Read the model definition and answer for the solid it produces. Units are mm, in the model's axes. Face numbers are marked on the shaded views. Coordinates: 2 decimals unless noted, no trailing zeros. Write each loop counter-clockwise with the first axis right and the second up, starting at its lowest first coordinate (ties: lowest second). Pieces come first, ordered by that corner, then holes. Notation, with made-up numbers: (33.25, 28) -> (54.25, 28) arc R21 ccw to (54.25, 66) -> close; hole circle Ø7 at (75.25, -40). An arc over 180 degrees is marked (long way). Answer in a Markdown table with one row per item. Add a question column.
Item 1: Section A-A on x = 0 is taken. Write down the section's boundary in (y, z).
Item 2: Given pin 1 Ø1 at (x, z) = (-9.5, 11) entering from +Y; pin 2 Ø3.5 at (x, y) = (0, -8) entering from +Z; pin 3 Ø5 at (x, z) = (-3, 8) entering from -Y, each flat-ended and moving along its own axis, determine where each tip first touches the part or whether it passes through.
Item 3: Straight lines are drawn through the part: line 1 (Y direction, x = 0, z = 11); line 2 (X direction, y = -9, z = 13); line 3 (Y direction, x = -13, z = 11). For each, find the intervals that lie inside material, in ascending order. Write a range as from..to.
Item 4: For a pull along X with two mould halves and no side action, classify the marked faces 1, 2 and 3 as +X half, -X half, draft (parallel to the pull), parting line (faces both ways), or undercut.
Item 5: Section B-B on z = 8.5 is taken. Write down the section's boundary in (x, y), then the cut area to 3 significant figures.
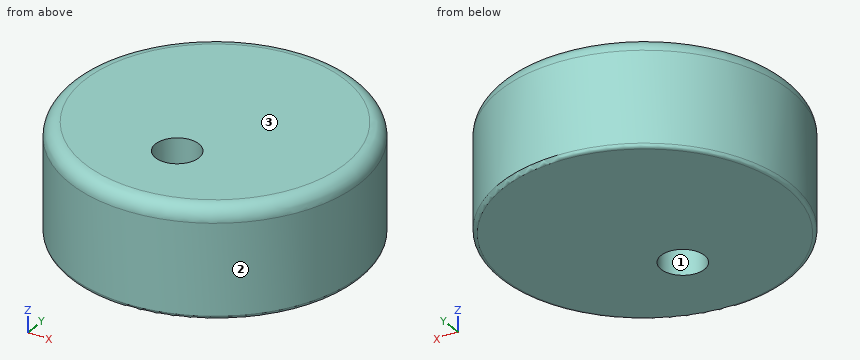
```python
from build123d import *

# Parameters (mm, degrees)
SKETCH1_R           = 20
BOSS_EXTRUDE1_DEPTH = 15
SKETCH2_R           = 3
CUT_EXTRUDE1_DEPTH  = 16
FILLET1_R           = 2
FILLET2_R           = 0.5


with BuildPart() as part:
    # Sketch1 → Boss-Extrude1 (new body)
    with BuildSketch(Plane.XY):
        Circle(SKETCH1_R)
    extrude(amount=BOSS_EXTRUDE1_DEPTH)

    # Sketch2 → Cut-Extrude1 (cut, through all)
    with BuildSketch(Plane.XY.offset(15)):
        with Locations((0, -8)):
            Circle(SKETCH2_R)
    extrude(amount=-CUT_EXTRUDE1_DEPTH, mode=Mode.SUBTRACT)

    # Fillet1
    fillet1_edges = [part.edges().sort_by_distance(p)[0] for p in [
        (-20, 0, 15),
    ]]
    fillet(fillet1_edges, radius=FILLET1_R)

    # Fillet2
    fillet2_edges = [part.edges().sort_by_distance(p)[0] for p in [
        (-20, 0, 0),
    ]]
    fillet(fillet2_edges, radius=FILLET2_R)


solid = part.part
```
Results below:
| question | item | result |
|---|---|---|
| 1 | outline | (-20, 0.5) arc R0.5 ccw to (-19.5, 0) -> (-11, 0) -> (-11, 15) -> (-18, 15) arc R2 ccw to (-20, 13) -> close; (-5, 0) -> (19.5, 0) arc R0.5 ccw to (20, 0.5) -> (20, 13) arc R2 ccw to (18, 15) -> (-5, 15) -> close |
| 2 | pin 1 | stops at y = 17.86 |
| 2 | pin 2 | passes through |
| 2 | pin 3 | stops at y = -19.99 |
| 3 | line 1 | y = -20..-11, -5..20 |
| 3 | line 2 | x = -17.86..-2.83, 2.83..17.86 |
| 3 | line 3 | y = -15.2..15.2 |
| 4 | face 1 | undercut |
| 4 | face 2 | parting line |
| 4 | face 3 | draft |
| 5 | outline | circle Ø40 at (0, 0); hole circle Ø6 at (0, -8) |
| 5 | area | 1,230 mm2 |
